```python
from build123d import *

# Parameters (mm, degrees)
BOX014_W     = 2
BOX014_H     = 35
BOX014_DEPTH = 16
BOX015_W     = 2
BOX015_H     = 35
BOX015_DEPTH = 16
BOX017_W     = 21
BOX017_H     = 2
BOX017_DEPTH = 16
FILLET012_R  = 2


with BuildPart() as cubo013:
    # Box014 → Box014 (new body)
    with BuildSketch(Plane(origin=(29, 29, -46), x_dir=(1, 0, 0), z_dir=(0, 0, 1))):
        with Locations((1, 17.5)):
            Rectangle(BOX014_W, BOX014_H)
    extrude(amount=BOX014_DEPTH)


with BuildPart() as cubo014:
    # Box015 → Box015 (new body)
    with BuildSketch(Plane(origin=(48, 29, -46), x_dir=(1, 0, 0), z_dir=(0, 0, 1))):
        with Locations((1, 17.5)):
            Rectangle(BOX015_W, BOX015_H)
    extrude(amount=BOX015_DEPTH)


with BuildPart() as fillet012:
    # Box017 → Box017 (new body)
    with BuildSketch(Plane(origin=(29, 62, -46), x_dir=(1, 0, 0), z_dir=(0, 0, 1))):
        with Locations((10.5, 1)):
            Rectangle(BOX017_W, BOX017_H)
    extrude(amount=BOX017_DEPTH)

    # Fusion: union Cubo013, Cubo014
    add(cubo013.part)
    add(cubo014.part)

    # Fillet012
    fillet012_edges = [fillet012.edges().sort_by_distance(p)[0] for p in [
        (30, 29, -30),
        (49, 29, -30),
        (29, 64, -38),
        (50, 64, -38),
    ]]
    fillet(fillet012_edges, radius=FILLET012_R)


with BuildPart() as fillet012_1:
    # Fillet012 placement: moved
    add(fillet012.part.moved(Location((0, -13, 3))))


solid = fillet012_1.part
```
Can you work these out from the model? Positions are in its coordinate system, mm. A direction names the side the tool comes from. Give positions to 0.01 mm unless a question says otherwise; leave off trailing zeros. Write each loop counter-clockwise with the first axis right and the second up, starting at its lowest first coordinate (ties: lowest second). Pieces come first, ordered by that corner, then holes. Notation, with made-up numbers: (12.25, 41) -> (31.25, 41) arc R22 cw to (31.25, 58) -> close; hole circle Ø2 at (-30.5, -38.75). An arc over 180 degrees is marked (long way). Write item = value, one per line.
(1) For faces 1 (the face through (31, 32, -35)), 2 (the face through (39, 51, -35)), which set-ups out of +Z, -Z, +X, -X, +Y, -Y let a thin tool reach every point of the face, with its end or its side?
Worked out:
face_1 = +Z, -Z, -Y
face_2 = +Z, -Z, +X, -X, +Y
(2) I'm going to push a flat-ended pin straight in: P1, Ø1.5, axis at x = 38, z = -33, coming from the -Y side. Where does the tip first touch, or does it pass through?
Worked out:
P1 = 49
(3) Thinking about a two-plate mould opening in X: for faces 3 (the face through (29, 32, -35)), 4 (the face through (30, 37, -43)), 5 (the face through (39, 49, -35)), 6 (the face through (48, 32, -35)), which applies, released by +X, released by -X, zero draft, split by the parting line, or undercut?
Worked out:
face_3 = released by -X
face_4 = zero draft
face_5 = undercut
face_6 = undercut
(4) Suppose I cut it at A-A on y = 24. Write out the boundary of the cut face in (x, z), then the cut area to 3 significant figures.
Worked out:
outline = (29, -43) -> (31, -43) -> (31, -27) -> (29, -27) -> close; (48, -43) -> (50, -43) -> (50, -27) -> (48, -27) -> close
area = 64.0 mm^2
(5) Suppose I cut it at C-C on x = 37.25. Write out the boundary of the cut face in (y, z).
Worked out:
outline = (49, -43) -> (51, -43) -> (51, -27) -> (49, -27) -> close
(6) Suppose I cut it at D-D on z = -27.75. Write out the boundary of the cut face in (x, y).
Worked out:
outline = (29, 16.44) -> (31, 16.44) -> (31, 49) -> (48, 49) -> (48, 16.44) -> (50, 16.44) -> (50, 49) arc R2 ccw to (48, 51) -> (31, 51) arc R2 ccw to (29, 49) -> close
(7) Suppose I cut it at B-B on z = -38. Write out the boundary of the cut face in (x, y).
Worked out:
outline = (29, 16) -> (31, 16) -> (31, 49) -> (48, 49) -> (48, 16) -> (50, 16) -> (50, 49) arc R2 ccw to (48, 51) -> (31, 51) arc R2 ccw to (29, 49) -> close
(8) I need wall thicknesses on probe 1 along X at (y, z) = (25.5, -35.5); probe 2 along Y at (x, z) = (34.25, -28.5). Which ranges of each line are inside material? Lowest first, please. Write a range as from..to.
Worked out:
probe_1 = 29..31, 48..50
probe_2 = 49..51
